```python
from build123d import *

# Parameters (mm, degrees)
SKIZZE1_W                                           = 100
SKIZZE1_H                                           = 50
AUFSATZ_LINEAR_AUSTRAGEN1_DEPTH                     = 100
KERNLOCH_F_R_M8_HELICOIL1_D                         = 8.3
KERNLOCH_F_R_M8_HELICOIL1_DEPTH                     = 20
KERNLOCH_F_R_M8_HELICOIL1_TIP                       = 2.493571569
STIRNSENKUNG_F_R_M8_SENKSCHRAUBE_KOPF_B_D           = 9
STIRNSENKUNG_F_R_M8_SENKSCHRAUBE_KOPF_B_CBORE_D     = 15
STIRNSENKUNG_F_R_M8_SENKSCHRAUBE_KOPF_B_CBORE_DEPTH = 116
KERNLOCH_F_R_M8_HELICOIL2_D                         = 8.3
KERNLOCH_F_R_M8_HELICOIL2_DEPTH                     = 20
KERNLOCH_F_R_M8_HELICOIL2_TIP                       = 2.493571569


with BuildPart() as part:
    # Skizze1 → Aufsatz-Linear austragen1 (new body)
    with BuildSketch(Plane.XY):
        Rectangle(SKIZZE1_W, SKIZZE1_H)
    extrude(amount=AUFSATZ_LINEAR_AUSTRAGEN1_DEPTH)

    # Kernloch für M8 Helicoil1
    with Locations(Plane(origin=(0, 25, 0), x_dir=(1, 0, 0), z_dir=(0, 1, 0))):
        with Locations((35, -85), (-35, -15)):
            Hole(KERNLOCH_F_R_M8_HELICOIL1_D / 2, depth=KERNLOCH_F_R_M8_HELICOIL1_DEPTH)
            with Locations((0, 0, -(KERNLOCH_F_R_M8_HELICOIL1_DEPTH + KERNLOCH_F_R_M8_HELICOIL1_TIP / 2))):  # 118° drill point
                Cone(0, KERNLOCH_F_R_M8_HELICOIL1_D / 2, KERNLOCH_F_R_M8_HELICOIL1_TIP, mode=Mode.SUBTRACT)

    # Stirnsenkung für M8 Senkschraube (Kopf Button)1 (through all)
    with Locations(Plane.XY.offset(100)):
        with Locations((4.444e-06, 5)):
            CounterBoreHole(STIRNSENKUNG_F_R_M8_SENKSCHRAUBE_KOPF_B_D / 2, STIRNSENKUNG_F_R_M8_SENKSCHRAUBE_KOPF_B_CBORE_D / 2, STIRNSENKUNG_F_R_M8_SENKSCHRAUBE_KOPF_B_CBORE_DEPTH)

    # Kernloch für M8 Helicoil2
    with Locations(Plane(origin=(0, 0, 0), x_dir=(-1, 0, 0), z_dir=(0, 0, -1))):
        with Locations((19.230769231, 5.769226325)):
            Hole(KERNLOCH_F_R_M8_HELICOIL2_D / 2, depth=KERNLOCH_F_R_M8_HELICOIL2_DEPTH)
            with Locations((0, 0, -(KERNLOCH_F_R_M8_HELICOIL2_DEPTH + KERNLOCH_F_R_M8_HELICOIL2_TIP / 2))):  # 118° drill point
                Cone(0, KERNLOCH_F_R_M8_HELICOIL2_D / 2, KERNLOCH_F_R_M8_HELICOIL2_TIP, mode=Mode.SUBTRACT)


solid = part.part
```
Check sheet for the modelled part. Datum: model origin and axes. Units: mm. A direction names the side the tool comes from. Coordinates: 2 decimals unless noted, no trailing zeros. Loops run counter-clockwise (first coordinate to the right, second up) from the corner with the lowest first, then second, coordinate; pieces in that order, holes last.
1) Access from +Z, -Z, +X, -X, +Y, -Y to the whole of each face (thin tool, end or side, straight path). Record for faces 1 (the face through (-38.834, 14.86, 16.589)), 2 (the face through (-17.316, 2.087, 10.14)), 3 (the face through (-1, -25, 49)).
2) Material ranges on probe 1 along Z at (x, y) = (35, 13); probe 2 along X at (y, z) = (13, 85); probe 3 along Z at (x, y) = (-35, 9), recorded low to high.
3) Release check for a two-part mould opening along Z. For faces 4 (the face through (50, 0, 49)), 5 (the face through (32.77, 14.86, 81.5)), 6 (the face through (-19.075, 5.066, 22.061)), 7 (the face through (35.39, 2.94, 84.39)) record: released by +Z, released by -Z, zero draft, split by the parting line, or undercut.
4) Sectioned sample at B-B (z = 61.5). Record the boundary of the cut face in (x, y).
5) Sectioned sample at A-A (y = -1). Record the boundary of the cut face in (x, z), and give its area (3 significant figures).
6) Gauge pin test, flat end, axial feed: pin 1 (9 mm diameter, centred on x = 0, y = 5, fed in from +Z). Record the tip position at first contact, or that the pin passes through.
Check sheet entries:
1. face 1: +Y
1. face 2: -Z
1. face 3: +Z, -Z, +X, -X, -Y
2. probe 1: z = 0 to 80.85, 89.15 to 100
2. probe 2: x = -50 to 30.85, 39.15 to 50
2. probe 3: z = 0 to 10.85, 19.15 to 100
3. face 4: zero draft
3. face 5: undercut
3. face 6: released by -Z
3. face 7: undercut
4. outline: (-50, -25) - (50, -25) - (50, 25) - (-50, 25) - close; hole circle Ø15 at (0, 5)
5. outline: (-50, 0) - (-4.5, 0) - (-4.5, 100) - (-50, 100) - close; (4.5, 0) - (50, 0) - (50, 100) - (4.5, 100) - close
5. area: 9,100 mm2
6. pin 1: passes through
